```python
from build123d import *

# Parameters (mm, degrees)
F0_W     = 1156
F0_H     = 706
F0_W_2   = 1150
F0_H_2   = 700
F1_DEPTH = 150
F2_W     = 5
F2_H     = 706
F3_DEPTH = 1153


with BuildPart() as f1:
    # F0 (on Front) → F1 (new body)
    with BuildSketch(Plane.XZ):
        with Locations((503.755269, -311.657544)):
            Rectangle(F0_W, F0_H)
        with Locations((503.755269, -311.657544)):
            Rectangle(F0_W_2, F0_H_2, mode=Mode.SUBTRACT)
    extrude(amount=F1_DEPTH)

    # F2 (on face) → F3 (join, through all)
    with BuildSketch(Plane(origin=(-74.244731, 0, 0), x_dir=(0, -1, 0), z_dir=(-1, 0, 0))):
        with Locations((2.5, -311.657544)):
            Rectangle(F2_W, F2_H)
    extrude(amount=-F3_DEPTH)


solid = f1.part
```
Source: CAD feature listing. Evaluate the final solid. Frame: model axes, mm. A direction names the side the tool comes from. Round coordinates to 2 decimals unless told otherwise and drop trailing zeros. Order: outer loops, then holes, each group sorted by start corner. A loop starts at its lowest first (then second) coordinate and runs counter-clockwise, first axis right, second up. Notation, with made-up numbers: (85, -15.5) -> (116, -15.5) arc R28 ccw to (116, 12.5) -> close; hole circle Ø9 at (-8.75, 28.25). An arc over 180 degrees is marked (long way). One line per item, written item: value. Start each with the question number.
Q1. Section query C-C (z = -279). Return the cut outline in (x, y).
Q2. Material intervals for probe 1 along Z at (x, y) = (214.5, -101); probe 2 along X at (y, z) = (-10.5, -5); probe 3 along Y at (x, z) = (646.5, -620.5), sorted ascending.
Q3. Section query A-A (y = -48). Return the cut outline in (x, z), plus the area to 3 significant figures.
Q4. Section query B-B (x = 260.5). Return the cut outline in (y, z).
Q5. Pin query (flat end, axial travel): pin 1 (1.5 mm diameter, centred on x = 212.5, z = -131, fed in from -Y). Return the tip coordinate at first contact, or that it passes through.
Q6. Draft query along Z for faces 3 (the flat face through (496, -74, 41.342)), 4 (the flat face through (496, -76, 38.342)), 5 (the flat face through (-74.245, -74, -317)). Return one class per face: pulls with the +Z half, pulls with the -Z half, needs draft (parallel to the pull), parting line crosses it, or undercut.
Q7. Access query for faces 1 (the flat face through (-71.245, -76, -317)), 2 (the flat face through (496, -74, -664.658)). Directions: +Z, -Z, +X, -X, +Y, -Y. A direction counts if a zero-diameter tool reaches every point of the face in a straight line with its end or side. Return the directions, or none.
Findings below:
1. outline: (-74.24, -150) -> (-71.24, -150) -> (-71.24, -5) -> (1078.76, -5) -> (1078.76, -150) -> (1081.76, -150) -> (1081.76, 0) -> (-74.24, 0) -> close
2. probe 1: -664.66 to -661.66, 38.34 to 41.34
2. probe 2: -74.24 to -71.24, 1078.76 to 1081.76
2. probe 3: -5 to 0
3. outline: (-74.24, -664.66) -> (1081.76, -664.66) -> (1081.76, 41.34) -> (-74.24, 41.34) -> close; hole (-71.24, -661.66) -> (1078.76, -661.66) -> (1078.76, 38.34) -> (-71.24, 38.34) -> close
3. area: 11,100 mm²
4. outline: (-150, -664.66) -> (0, -664.66) -> (0, 41.34) -> (-150, 41.34) -> (-150, 38.34) -> (-5, 38.34) -> (-5, -661.66) -> (-150, -661.66) -> close
5. pin 1: y = -5
6. face 3: pulls with the +Z half
6. face 4: undercut
6. face 5: needs draft
7. face 1: -Y
7. face 2: -Z, +X, -X, +Y, -Y
